```python
from build123d import *

# Parameters (mm, degrees)
F1_DEPTH = 20.000011


with BuildPart() as f1:
    # F0 (on Front) → F1 (new body)
    with BuildSketch(Plane.XZ):
        with BuildLine():
            ThreePointArc((-3.271326, 21.764202), (-14.359396, -16.679023), (22.008682, 0))
            ThreePointArc((22.008682, 0), (15.704163, 15.419512), (0.402541, 22.005))
            ThreePointArc((0.402541, 22.005), (-1.439437, 21.961559), (-3.271326, 21.764202))
        make_face()
        with BuildLine():
            ThreePointArc((-3.271326, 21.764202), (-1.439437, 21.961559), (0.402541, 22.005))
            ThreePointArc((0.402541, 22.005), (0.294678, 23.039922), (0, 24.037851))
            ThreePointArc((0, 24.037851), (-0.516199, 25.054794), (-1.207822, 25.961598))
            ThreePointArc((-1.207822, 25.961598), (-1.455449, 25.953355), (-1.703043, 25.944164))
            ThreePointArc((-1.703043, 25.944164), (-1.943324, 25.927273), (-2.183439, 25.908157))
            ThreePointArc((-2.183439, 25.908157), (-2.755717, 24.913941), (-3.137569, 23.832204))
            ThreePointArc((-3.137569, 23.832204), (-3.299471, 22.804349), (-3.271326, 21.764202))
        make_face()
    extrude(amount=F1_DEPTH)


solid = f1.part
```
Geometry: final body of the model. Coordinates: model frame, mm. Give positions to 0.01 mm unless a question says otherwise; leave off trailing zeros. Loops run counter-clockwise (first coordinate to the right, second up) from the corner with the lowest first, then second, coordinate; pieces in that order, holes last. Notation, with made-up numbers: (59, -7.75) - (69, -7.75) arc R13 cw to (69, 16.25) - close; hole circle Ø10 at (65.25, -7.75). An arc over 180 degrees is marked (long way). Answer as CSV lines item,"result". Start each with the question number.
(1) Section query B-B (x = 8.5). Output: boundary loops of the cut face in (y, z).
(2) Section query A-A (y = -7.5). Output: boundary loops of the cut face in (x, z) (3 decimals), and give its area (3 significant figures).
(3) Mould query, pull axis Z, two halves, no side actions, for faces 1 (the face through (-3.3, -9.9, 22.8)), 2 (the face through (-0.508, -9.86, 25.041)), 3 (the face through (0, -20, 2)). Classes: +Z half, -Z half, draft (parallel to the pull), parting line (faces both ways), or undercut.
(4) Section query C-C (z = -16.5). Output: boundary loops of the cut face in (x, y).
(5) Pin query (flat end, axial travel): P1, Ø5, axis at x = 10, y = -11, coming from the +Z side; P2, Ø5, axis at y = -5.5, z = -15.5, coming from the -X side; P3, Ø10, axis at x = 16.5, y = -4.5, coming from the +Z side. Return the tip coordinate at first contact, or that it passes through.
(6) Ray query, line 1 along X through (y, z) = (-12.75, 0.5); line 2 along Z through (x, y) = (-4.5, -4.25). Return the intervals inside material, ascending. Write a range as [from, to].
Worked answers:
1,outline,"(-20, -20.3) - (0, -20.3) - (0, 20.3) - (-20, 20.3) - close"
2,outline,"(-3.271, 21.764) arc R22.009 ccw (long way) to (0.403, 22.005) arc R5.685 ccw to (0, 24.038) arc R6.279 ccw to (-1.208, 25.962) arc R64.715 ccw to (-1.703, 25.944) arc R26.004 ccw to (-2.183, 25.908) arc R6.279 ccw to (-3.138, 23.832) arc R5.685 ccw to start"
2,area,"1,530 mm^2"
3,face 1,"undercut"
3,face 2,"+Z half"
3,face 3,"draft"
4,outline,"(-14.56, -20) - (14.56, -20) - (14.56, 0) - (-14.56, 0) - close"
5,P1,"stops at z = 20.69"
5,P2,"stops at x = -17.76"
5,P3,"stops at z = 18.77"
6,line 1,"x = [-22, 22]"
6,line 2,"z = [-21.54, 21.54]"
